The listing builds one solid part. Answer for the finished solid, in the listing's coordinates (mm). A direction names the side the tool comes from. Give positions to 0.01 mm unless a question says otherwise; leave off trailing zeros. Write each loop counter-clockwise with the first axis right and the second up, starting at its lowest first coordinate (ties: lowest second). Pieces come first, ordered by that corner, then holes. Notation, with made-up numbers: (-16, 84) - (37, 84) arc R30 ccw to (37, 123) - close; hole circle Ø4 at (73.25, -5). An arc over 180 degrees is marked (long way). Use a Markdown table: item, result. Add a question column.
Autodesk Inventor part; units mm, degrees
ref_plane "YZ Plane" through (0, 0, 0) normal (1, 0, 0) x (0, 1, 0)
ref_plane "XZ Plane" through (0, 0, 0) normal (0, 1, 0) x (-1, 0, 0)
ref_plane "XY Plane" through (0, 0, 0) normal (0, 0, 1) x (1, 0, 0)
sketch "Sketch1" plane through (0, 0, 0) normal (0, 0, 1) x (1, 0, 0)
  line L0 (0, 0) -> (100, 0)
  line L1 (100, 0) -> (100, 80) construction
  line L2 (100, 80) -> (0, 80)
  line L3 (0, 80) -> (0, 0)
  line L4 (100, 70) -> (90, 80)
  line L5 (100, 10) -> (90, 0)
  line L6 (100, 70) -> (100, 10)
  dimension "d0" = 100
  dimension "d1" = 80
  dimension "d23" = 10
  dimension "d24" = 10
  dimension "d25" = 10
  dimension "d26" = 10
extrude "Extrusion1" add sketch "Sketch1" along normal blind 40
sketch "Sketch4" plane through (0, 0, 0) normal (0, 0, -1) x (-1, 0, 0)
  line L0 (-90, 80) -> (0, 80)
  line L1 (0, 0) -> (-90, 0)
  line L2 (-100, 70) -> (-90, 80)
  line L3 (-100, 10) -> (-100, 70)
  line L4 (-90, 0) -> (-100, 10)
  line L5 (0, 75) -> (-87.9289, 75)
  line L6 (-87.9289, 75) -> (-95, 67.9289)
  line L7 (-95, 67.9289) -> (-95, 12.0711)
  line L8 (-95, 12.0711) -> (-87.9289, 5)
  line L9 (-87.9289, 5) -> (0, 5)
  line L10 (0, 75) -> (0, 5)
  line L11 (0, 80) -> (0, 0)
  dimension "d27" = 5
extrude "Extrusion4" cut sketch "Sketch4" against normal blind 35 contours L10 L9 L8 L7 L6 L5
sketch "Sketch5" plane through (0, 0, 40) normal (-1, 0, 0) x (0, 0, 1)
  line L0 (0, 0) -> (0, 80)
  line L1 (-40, 5) -> (-40, 75)
  line L2 (0, 80) -> (-40, 80)
  line L3 (-40, 80) -> (-40, 70)
  line L4 (-40, 70) -> (0, 70)
  line L5 (0, 70) -> (0, 80)
  line L6 (0, 80) -> (-10, 80)
  line L7 (-10, 80) -> (-10, 50)
  line L8 (-10, 50) -> (0, 50)
  line L9 (0, 50) -> (0, 80)
  line L10 (-40, 0) -> (0, 0)
  dimension "d15" = 10
  dimension "d16" = 10
  dimension "d17" = 50
extrude "Extrusion5" add sketch "Sketch5" against normal blind 5
sketch "Sketch6" plane through (100, 10, 0) normal (1, 0, 0) x (0, 0, -1)
  circle A0 centre (0, 30) radius 16
  line L0 (0, 0) -> (0, 60)
  dimension "d20" = 32
extrude "Extrusion6" cut sketch "Sketch6" against normal through all
sketch "Sketch7" plane through (0, 0, 35) normal (0, 0, -1) x (-1, 0, 0)
  line L0 (-87.9289, 75) -> (-5, 75)
  line L1 (0, 5) -> (-87.9289, 5)
  line L2 (-74, 75) -> (-69, 75)
  line L3 (-69, 75) -> (-69, 5)
  line L4 (-69, 5) -> (-74, 5)
  line L5 (-74, 5) -> (-74, 75)
  line L6 (-95, 56) -> (-95, 67.9289)
  line L7 (-24, 75) -> (-19, 75)
  line L8 (-19, 75) -> (-19, 5)
  line L9 (-19, 5) -> (-24, 5)
  line L10 (-24, 5) -> (-24, 75)
  line L11 (-69, 67.5) -> (-24, 67.5)
  line L12 (-24, 67.5) -> (-24, 62.5)
  line L13 (-24, 62.5) -> (-69, 62.5)
  line L14 (-69, 62.5) -> (-69, 67.5)
  line L15 (-69, 17.5) -> (-24, 17.5)
  line L16 (-24, 17.5) -> (-24, 12.5)
  line L17 (-24, 12.5) -> (-69, 12.5)
  line L18 (-69, 12.5) -> (-69, 17.5)
  line L19 (-46.5, 67.5) -> (-46.5, 12.5) construction
  point P0 (0, 0)
  point P1 (-46.5, 40)
  point P2 (-69, 40)
  dimension "d28" = 5
  dimension "d29" = 21
  dimension "d30" = 5
  dimension "d31" = 45
  dimension "d32" = 5
  dimension "d33" = 5
  dimension "d34" = 45
extrude "Extrusion7" add sketch "Sketch7" along normal blind 35 contours L0 L3 L1 L5 | L0 L8 L1 L10 | L11 L10 L13 L3 | L3 L15 L10 L17
sketch "Sketch8" plane through (0, 0, 0) normal (0, 0, -1) x (-1, 0, 0)
  line L0 (-19, 5) -> (-19, 75)
  line L1 (-69, 17.5) -> (-24, 17.5)
  line L2 (-19, 5) -> (-42, 5)
  line L3 (-42, 5) -> (-42, 17.5)
  line L4 (-42, 17.5) -> (-19, 17.5)
  line L5 (-19, 17.5) -> (-19, 5)
  point P0 (0, 0)
  dimension "d37" = 23
extrude "Extrusion8" cut sketch "Sketch8" against normal blind 10
sketch "Sketch9" plane through (69, 17.5, 35) normal (-1, 0, 0) x (0, 0, 1)
  line L0 (-35, 0) -> (-35, 45)
  circle A0 centre (-35, 22.5) radius 2.75
  line L1 (-50.5, 7) -> (-19.5, 7) construction
  line L2 (-19.5, 7) -> (-19.5, 38) construction
  line L3 (-19.5, 38) -> (-50.5, 38) construction
  line L4 (-50.5, 38) -> (-50.5, 7) construction
  line L5 (-50.5, 7) -> (-19.5, 38) construction
  line L6 (-19.5, 7) -> (-50.5, 38) construction
  circle A1 centre (-19.5, 38) radius 1.5
  circle A2 centre (-19.5, 7) radius 1.5
  point P0 (-35, -17.5)
  dimension "d40" = 5.5
  dimension "d41" = 31
  dimension "d42" = 31
  dimension "d43" = 3
  dimension "d44" = 3
extrude "Extrusion9" cut sketch "Sketch9" against normal through all
sketch "Sketch10" plane through (0, 0, 35) normal (0, 0, -1) x (-1, 0, 0)
  line L0 (-30, 59.5) -> (-33, 59.5)
  line L1 (-33, 59.5) -> (-33, 20.5)
  line L2 (-33, 20.5) -> (-30, 20.5)
  line L3 (-30, 20.5) -> (-30, 59.5)
  line L4 (-24, 62.5) -> (-24, 17.5)
  line L5 (-69, 62.5) -> (-24, 62.5)
  line L6 (-24, 17.5) -> (-19, 17.5)
  line L7 (-36, 59.5) -> (-39, 59.5)
  line L8 (-39, 59.5) -> (-39, 20.5)
  line L9 (-39, 20.5) -> (-36, 20.5)
  line L10 (-36, 20.5) -> (-36, 59.5)
  line L11 (-42, 59.5) -> (-45, 59.5)
  line L12 (-45, 59.5) -> (-45, 20.5)
  line L13 (-45, 20.5) -> (-42, 20.5)
  line L14 (-42, 20.5) -> (-42, 59.5)
  line L15 (-48, 59.5) -> (-51, 59.5)
  line L16 (-51, 59.5) -> (-51, 20.5)
  line L17 (-51, 20.5) -> (-48, 20.5)
  line L18 (-48, 20.5) -> (-48, 59.5)
  line L19 (-54, 59.5) -> (-57, 59.5)
  line L20 (-57, 59.5) -> (-57, 20.5)
  line L21 (-57, 20.5) -> (-54, 20.5)
  line L22 (-54, 20.5) -> (-54, 59.5)
  line L23 (-60, 59.5) -> (-63, 59.5)
  line L24 (-63, 59.5) -> (-63, 20.5)
  line L25 (-63, 20.5) -> (-60, 20.5)
  line L26 (-60, 20.5) -> (-60, 59.5)
  point P0 (0, 0)
  dimension "d47" = 3
  dimension "d49" = 6
  dimension "d50" = 3
  dimension "d51" = 3
  dimension "d54" = 6
extrude "Extrusion10" cut sketch "Sketch10" against normal through all
sketch "Sketch11" plane through (0, 0, 0) normal (0, -1, 0) x (1, 0, 0)
  circle A0 centre (45, 0) radius 6
  line L0 (0, 0) -> (90, 0)
  dimension "d61" = 12
extrude "Extrusion11" cut sketch "Sketch11" against normal blind 5
sketch "Sketch12" plane through (69, 17.5, 35) normal (-1, 0, 0) x (0, 0, 1)
  arc A0 (-35, 19.75) -> (-35, 25.25) centre (-35, 22.5) ccw
  circle A1 centre (-35, 22.5) radius 12.5
  point P0 (-35, -17.5)
  dimension "d64" = 25
extrude "Extrusion12" cut sketch "Sketch12" against normal blind 2
sketch "Sketch13" plane through (100, 10, 40) normal (1, 0, 0) x (0, 0, -1)
  arc A0 (40, 46) -> (40, 14) centre (40, 30) ccw
  circle A1 centre (17.5, 30) radius 2.5
  circle A2 centre (28.75, 10.5144) radius 2.5
  circle A3 centre (51.25, 10.5144) radius 2.5
  circle A4 centre (62.5, 30) radius 2.5
  circle A5 centre (51.25, 49.4856) radius 2.5
  circle A6 centre (28.75, 49.4856) radius 2.5
  point P0 (40, -10)
  dimension "d67" = 5
  dimension "d68" = 22.5
  dimension "d71" = 360
extrude "Extrusion13" cut sketch "Sketch13" against normal blind 10 contours A1 | A2 | A6
properties part number "FA002" material "ABS Plastic"
1. Consider L1, parallel to Y at x = 65, z = 28; L2, parallel to X at y = 26.5, z = 16.5; L3, parallel to Y at x = 30, z = 2.5. Determine where each line is inside the solid, lowest interval first. Write a range as [from, to].
2. The part is cut by section A-A (z = 22.5). Count the separate pieces of the cut face and the enclosed holes in it, and give its area (3 significant figures).
3. Which of the six approach directions +Z, -Z, +X, -X, +Y, -Y give full straight-line access (tool end or side, diameter ignored) to faces 1 (the flat face through (51, 40, 37)), 2 (the flat face through (28, 14, 10)), 3 (the flat face through (95, 40, 17))?
4. Given P1, Ø5, axis at y = 28.5, z = 14.5, coming from the -X side; P2, Ø2, axis at x = 39, y = 47, coming from the -Z side, each flat-ended and moving along its own axis, determine where each tip first touches the part or whether it passes through.
5. For a pull along Z with two mould halves and no side action, classify faces 4 (the flat face through (47, 9, 35)), 5 (the flat face through (39, 40, 37)), 6 (the cylindrical face through (97.535, 57.045, 11.792)) as released by +Z, released by -Z, zero draft, split by the parting line, or undercut.
6. The part is cut by section B-B (x = 83.5). Give the vertices of the cut face in (y, z).
Check values:
| question | item | result |
|---|---|---|
| 1 | L1 | y = [0, 5], [12.5, 17.5], [62.5, 67.5], [75, 80] |
| 1 | L2 | x = [19, 24], [69, 74], [95, 100] |
| 1 | L3 | y = [0, 5], [62.5, 67.5], [75, 80] |
| 2 | separate pieces | 1 |
| 2 | enclosed holes | 3 |
| 2 | area | 2,450 mm2 |
| 3 | face 1 | +Z, -Z |
| 3 | face 2 | -Z, -X |
| 3 | face 3 | -Z |
| 4 | P1 | stops at x = 19 |
| 4 | P2 | stops at z = 35 |
| 5 | face 4 | released by -Z |
| 5 | face 5 | zero draft |
| 5 | face 6 | undercut |
| 6 | outline | (0, 0) - (5, 0) - (5, 35) - (75, 35) - (75, 0) - (80, 0) - (80, 40) - (0, 40) - close |
